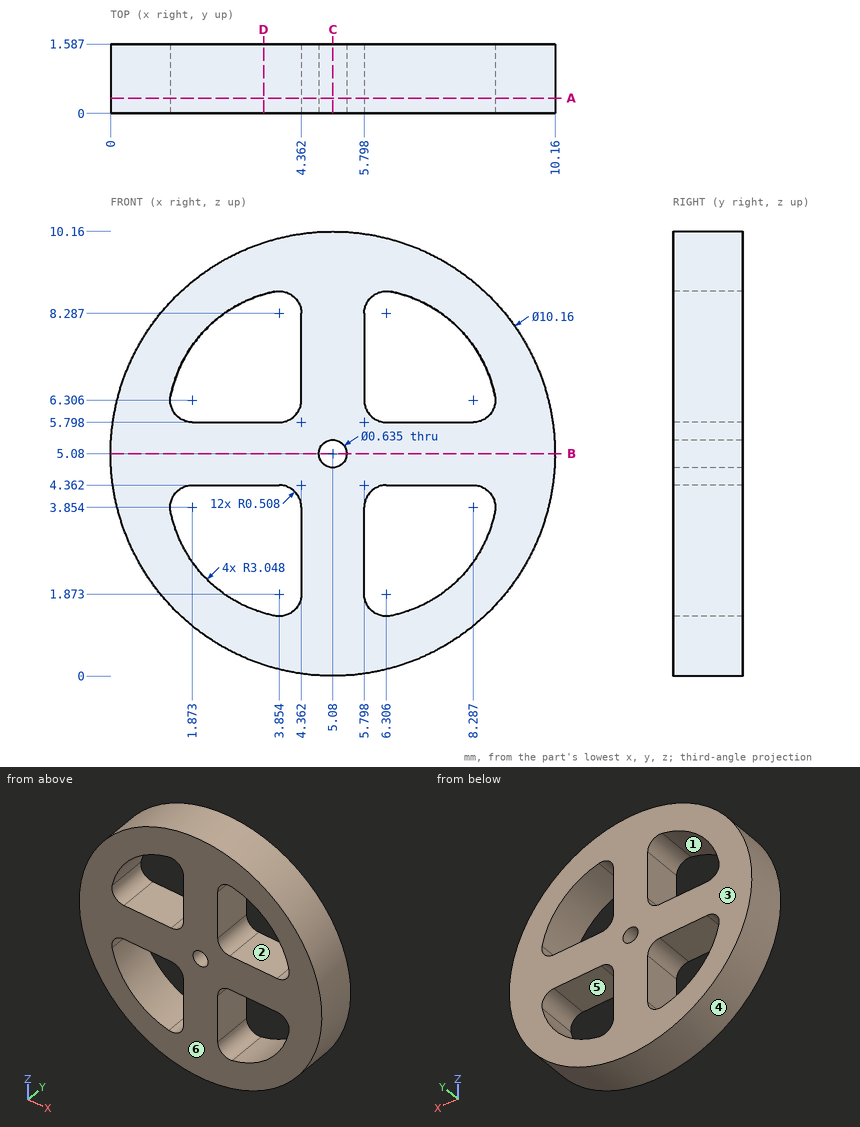
Source: three-view drawing plus pictorial views. Frame: mm from the lowest corner of the part. A direction names the side the tool comes from. Give positions to 0.01 mm unless a question says otherwise; leave off trailing zeros. Order: outer loops, then holes, each group sorted by start corner. A loop starts at its lowest first (then second) coordinate and runs counter-clockwise, first axis right, second up. Notation, with made-up numbers: (32.5, 25) -> (75.5, 25) arc R27 ccw to (75.5, 57) -> close; hole circle Ø4 at (-12, 87.5). An arc over 180 degrees is marked (long way). Write each question's results on one line, items separated by ' | '. Start each with the question number.
Item 1: Mould query, pull axis Z, two halves, no side actions, for the marked faces 1, 2, 3 and 4. Classes: pulls with the +Z half, pulls with the -Z half, needs draft (parallel to the pull), parting line crosses it, or undercut.
Item 2: Cut plane D-D on x = 3.5. Return the cut outline in (y, z).
Item 3: Cut plane B-B on z = 5.08. Return the cut outline in (x, y), then the cut area to 3 significant figures.
Item 4: Cut plane C-C on x = 5.08. Return the cut outline in (y, z), then the cut area to 3 significant figures.
Item 5: Contact query for flat-ended pins moving along their axis: P1, Ø0.5, axis at x = 2.5, y = 0.5, coming from the +Z side (1 decimal); P2, Ø0.5, axis at x = 2.5, y = 1, coming from the -Z side (1 decimal); P3, Ø0.5, axis at y = 1, z = 7, coming from the -X side; P4, Ø5, axis at x = 6.5, z = 5.5, coming from the -Y side. Output: stop coordinate, or through.
Item 6: Set-up query: the marked faces 5 and 6. Return all of +Z, -Z, +X, -X, +Y, -Y with unobstructed straight access to the full face (end or side cutting, diameter ignored); none if empty.
Item 7: Cut plane A-A on y = 0.35. Return the cut outline in (x, z) (1 decimal).
Item 8: Line query: line 1 (X direction, y = 0.9, z = 5.08); line 2 (X direction, y = 0.6, z = 3.25) (1 decimal); line 3 (Z direction, x = 7.75, y = 0.7). Output: solid intervals per line, ascending.
Established:
1) face 1: undercut | face 2: undercut | face 3: needs draft | face 4: parting line crosses it
2) outline: (0, 0.25) -> (1.59, 0.25) -> (1.59, 1.44) -> (0, 1.44) -> close; (0, 4.36) -> (1.59, 4.36) -> (1.59, 5.8) -> (0, 5.8) -> close; (0, 8.72) -> (1.59, 8.72) -> (1.59, 9.91) -> (0, 9.91) -> close
3) outline: (0, 0) -> (4.76, 0) -> (4.76, 1.59) -> (0, 1.59) -> close; (5.4, 0) -> (10.16, 0) -> (10.16, 1.59) -> (5.4, 1.59) -> close | area: 15.1 mm^2
4) outline: (0, 0) -> (1.59, 0) -> (1.59, 4.76) -> (0, 4.76) -> close; (0, 5.4) -> (1.59, 5.4) -> (1.59, 10.16) -> (0, 10.16) -> close | area: 15.1 mm^2
5) P1: z = 9.6 | P2: z = 0.6 | P3: x = 0.28 | P4: y = 0
6) face 5: +Y, -Y | face 6: +Z, -Z, +X, -X, -Y
7) outline: circle Ø10.2 at (5.1, 5.1); hole (1.4, 3.8) arc R3 ccw to (3.8, 1.4) arc R0.5 ccw to (4.4, 1.9) -> (4.4, 3.9) arc R0.5 ccw to (3.9, 4.4) -> (1.9, 4.4) arc R0.5 ccw to start; hole (1.4, 6.4) arc R0.5 ccw to (1.9, 5.8) -> (3.9, 5.8) arc R0.5 ccw to (4.4, 6.3) -> (4.4, 8.3) arc R0.5 ccw to (3.8, 8.8) arc R3 ccw to start; hole circle Ø0.6 at (5.1, 5.1); hole (5.8, 1.9) arc R0.5 ccw to (6.4, 1.4) arc R3 ccw to (8.8, 3.8) arc R0.5 ccw to (8.3, 4.4) -> (6.3, 4.4) arc R0.5 ccw to (5.8, 3.9) -> close; hole (5.8, 6.3) arc R0.5 ccw to (6.3, 5.8) -> (8.3, 5.8) arc R0.5 ccw to (8.8, 6.4) arc R3 ccw to (6.4, 8.8) arc R0.5 ccw to (5.8, 8.3) -> close
8) line 1: 0 to 4.76, 5.4 to 10.16 | line 2: 0.3 to 1.5, 4.4 to 5.8, 8.6 to 9.8 | line 3: 0.76 to 2.02, 4.36 to 5.8, 8.14 to 9.4
